Here's how the part is built. I have some questions about the finished solid (model axes, mm). A direction names the side the tool comes from. Round coordinates to 2 decimals unless told otherwise and drop trailing zeros. Loops run counter-clockwise (first coordinate to the right, second up) from the corner with the lowest first, then second, coordinate; pieces in that order, holes last. Notation, with made-up numbers: (57.25, 52) - (61.25, 52) arc R20 cw to (61.25, 57) - close; hole circle Ø8 at (-34, 23). An arc over 180 degrees is marked (long way). Answer as a JSON object with one key per item and string values. Group by question number.
1) Will these pins go through, and if not, where does the flat tip stop? P1, Ø1.5, axis at x = -3, y = 2.5, coming from the +Z side; P2, Ø1.8, axis at y = 6, z = -0.5, coming from the +X side; P3, Ø3, axis at x = 4, y = 8, coming from the -Z side; P4, Ø1.4, axis at x = -3.5, y = 8, coming from the +Z side.
2) I want a section at A-A, the plane x = 0. Please give me the cut outline in (y, z) (3 decimals).
3) I want a section at B-B, the plane y = 0. Please give me the cut outline in (x, z) (3 decimals), then the cut area to 3 significant figures.
4) Which directions (+Z, -Z, +X, -X, +Y, -Y) give clear straight access to the entire face, cutting with the end or side of a thin tool? Please do faces 4 (the face through (4, 7, 2.44)), 5 (the face through (-5.56, 7.11, -1.76)), 6 (the face through (-4.215, 0, 0)), 7 (the face through (-0.775, 1, 1)), 8 (the face through (-2.33, 7.11, 1.76)).
5) If I drill on line 1 along X through (y, z) = (6.25, -0.75); line 2 along Y through (x, z) = (-7, -3.5); line 3 along X through (y, z) = (3.25, -0.5) (3 decimals), over which ranges is the centre line in solid material (lowest first)? Write a range as [from, to].
6) If we mould it in two halves opening along Y, with no side actions, what happens to faces 1 (the face through (7.76, 4, 0)), 2 (the face through (0, 4.867, 0)), 3 (the face through (0.775, 1, 1))? For each: pulls with the +Y half, pulls with the -Y half, needs draft (parallel to the pull), parting line crosses it, or undercut.
7) I want a section at C-C, the plane z = 0. Please give me the cut outline in (x, y) (3 decimals), then the cut area to 3 significant figures.
8) I want a section at D-D, the plane z = 3.25. Please give me the cut outline in (x, y) (3 decimals).
from build123d import *

# Parameters (mm, degrees)
SKETCH1_R           = 1.155
BOSS_EXTRUDE1_DEPTH = 4.215
BOSS_EXTRUDE2_DEPTH = 0.775
BOSS_EXTRUDE3_DEPTH = 7.76
BOSS_EXTRUDE4_DEPTH = 4.55
CHAMFER1_SIZE       = 2.87
CHAMFER1_SIZE2      = 0.56


with BuildPart() as part:
    # Sketch1 → Boss-Extrude1 (new body)
    with BuildSketch(Plane(origin=(0, 0, 0), x_dir=(0, 0, -1), z_dir=(1, 0, 0))):
        Circle(SKETCH1_R)
    extrude(amount=BOSS_EXTRUDE1_DEPTH)

    # Sketch1_3 → Boss-Extrude2 (add)
    with BuildSketch(Plane(origin=(0, 0, 0), x_dir=(0, 0, -1), z_dir=(1, 0, 0))):
        with BuildLine():
            Line((-2.73, 2.737106893), (-2.73, 2.198209499))
            ThreePointArc((-2.73, 2.198209499), (0, -3.505), (2.73, 2.198209499))
            Line((2.73, 2.198209499), (2.73, 2.737106893))
            ThreePointArc((2.73, 2.737106893), (0, 3.6), (-2.73, 2.737106893))
        make_face()
    extrude(amount=BOSS_EXTRUDE2_DEPTH)

    # Sketch1_4 → Boss-Extrude3 (add)
    with BuildSketch(Plane(origin=(0, 0, 0), x_dir=(0, 0, -1), z_dir=(1, 0, 0))):
        with BuildLine():
            Line((-4.05, 2.737106893), (-2.73, 2.737106893))
            ThreePointArc((-2.73, 2.737106893), (0, 3.6), (2.73, 2.737106893))
            Line((2.73, 2.737106893), (4.05, 2.737106893))
            Line((4.05, 2.737106893), (4.05, 4.867106893))
            Line((4.05, 4.867106893), (-4.05, 4.867106893))
            Line((-4.05, 4.867106893), (-4.05, 2.737106893))
        make_face()
    extrude(amount=BOSS_EXTRUDE3_DEPTH)

    # Sketch2 → Boss-Extrude4 (add)
    with BuildSketch(Plane(origin=(0, 4.867106893, 0), x_dir=(1, 0, 0), z_dir=(0, 1, 0))):
        with BuildLine():
            Line((1.72, -1.333982369), (1.72, 1.333982369))
            ThreePointArc((1.72, 1.333982369), (2.322809893, 1.747089472), (2.555, 2.44))
            Line((2.555, 2.44), (5.335, 2.44))
            ThreePointArc((5.335, 2.44), (5.567190107, 1.747089472), (6.17, 1.333982369))
            Line((6.17, 1.333982369), (6.17, -1.333982369))
            ThreePointArc((6.17, -1.333982369), (5.567190107, -1.747089472), (5.335, -2.44))
            Line((5.335, -2.44), (2.555, -2.44))
            ThreePointArc((2.555, -2.44), (2.322809893, -1.747089472), (1.72, -1.333982369))
        make_face()
    extrude(amount=BOSS_EXTRUDE4_DEPTH)

    # Chamfer1
    chamfer1_edges = [part.edges().sort_by_distance(p)[0] for p in [
        (6.17, 9.417106893, 0),
    ]]
    chamfer1_side = [part.faces().sort_by_distance(p)[0] for p in [
        (6.17, 7.142106893, 0),
    ]]
    chamfer(chamfer1_edges, length=CHAMFER1_SIZE, length2=CHAMFER1_SIZE2, reference=chamfer1_side[0])

    # Mirror1: part across plane


with BuildPart() as part_1:
    add(part.part)
    add(part.part.mirror(Plane(origin=(0, 0, 0), x_dir=(0, 0, 1), z_dir=(1, 0, 0))))


solid = part_1.part
Outcome:
{
 "1": {"P1": "z = 4.05", "P2": "x = 6.17", "P3": "z = -2.44", "P4": "z = 2.44"},
 "2": {"outline": "(2.198, -2.73) - (2.737, -2.73) - (2.737, -4.05) - (4.867, -4.05) - (4.867, 4.05) - (2.737, 4.05) - (2.737, 2.73) - (2.198, 2.73) arc R3.505 ccw (long way) to start"},
 "3": {"outline": "(-4.215, -1.155) - (-0.775, -1.155) - (-0.775, -3.505) - (0.775, -3.505) - (0.775, -1.155) - (4.215, -1.155) - (4.215, 1.155) - (0.775, 1.155) - (0.775, 3.505) - (-0.775, 3.505) - (-0.775, 1.155) - (-4.215, 1.155) - close", "area": "26.8 mm^2"},
 "4": {"face 4": "+Z, +X, -X, +Y", "face 5": "-Z, -X, +Y", "face 6": "+Z, -Z, -X, -Y", "face 7": "-X", "face 8": "+Z, +Y"},
 "5": {"line 1": "[-6.17, -1.72], [1.72, 6.17]", "line 2": "[2.74, 4.87]", "line 3": "[-0.775, 0.775]"},
 "6": {"face 1": "needs draft", "face 2": "pulls with the +Y half", "face 3": "undercut"},
 "7": {"outline": "(-7.76, 3.6) - (-0.775, 3.6) - (-0.775, 1.155) - (-4.215, 1.155) - (-4.215, -1.155) - (-0.775, -1.155) - (-0.775, -3.505) - (0.775, -3.505) - (0.775, -1.155) - (4.215, -1.155) - (4.215, 1.155) - (0.775, 1.155) - (0.775, 3.6) - (7.76, 3.6) - (7.76, 4.867) - (6.17, 4.867) - (6.17, 6.547) - (5.61, 9.417) - (1.72, 9.417) - (1.72, 4.867) - (-1.72, 4.867) - (-1.72, 9.417) - (-5.61, 9.417) - (-6.17, 6.547) - (-6.17, 4.867) - (-7.76, 4.867) - close", "area": "85.5 mm^2"},
 "8": {"outline": "(-7.76, 2.737) - (7.76, 2.737) - (7.76, 4.867) - (-7.76, 4.867) - close; (-0.775, -1.312) - (0.775, -1.312) - (0.775, 1.312) - (-0.775, 1.312) - close"}
}
